Part print with two shaded views. Sizes in mm from the minimum x, y, z corner. Round coordinates to 2 decimals unless told otherwise and drop trailing zeros. Order: outer loops, then holes, each group sorted by start corner. A loop starts at its lowest first (then second) coordinate and runs counter-clockwise, first axis right, second up. Notation, with made-up numbers: (6.5, 40.25) - (45.5, 40.25) arc R16 ccw to (45.5, 51.25) - close; hole circle Ø6 at (65.25, 35). An arc over 180 degrees is marked (long way). Write item = value, one per line.
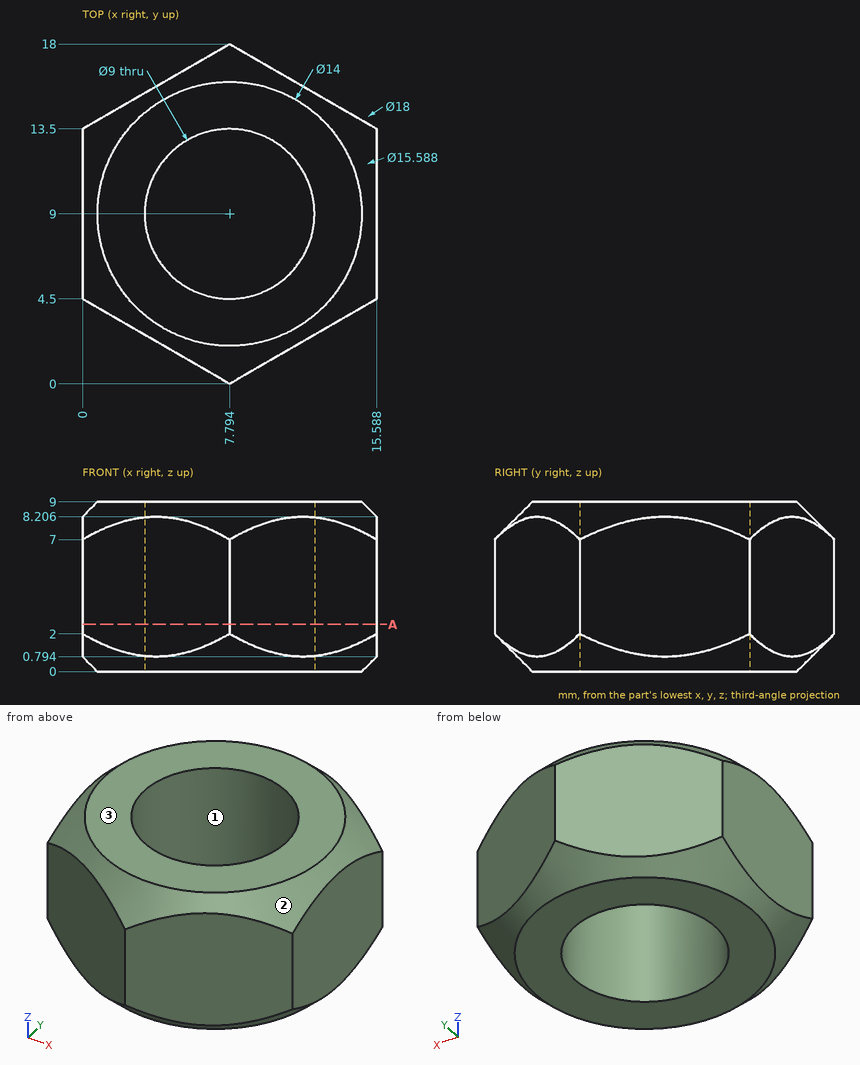
1) Mould opens along Y. For the marked faces 1, 2 and 3 say: +Y half, -Y half, draft (parallel to the pull), parting line (faces both ways), or undercut.
Conclusion:
face_1 = undercut
face_2 = parting line
face_3 = draft
2) Cut at A-A (z = 2.5). Write the cut outline in (x, y) (1 decimal).
Conclusion:
outline = (0, 4.5) - (7.8, 0) - (15.6, 4.5) - (15.6, 13.5) - (7.8, 18) - (0, 13.5) - close; hole circle Ø9 at (7.8, 9)
3) Flat gauge pins, fed straight in: pin 1 Ø1 at (x, z) = (2, 7) entering from -Y; pin 2 Ø2 at (y, z) = (2, 3.5) entering from -X; pin 3 Ø1.5 at (x, z) = (7.5, 1) entering from +Y (1 decimal). Where does each tip first touch, or does it go through?
Conclusion:
pin_1 = 3.06
pin_2 = 2.6
pin_3 = 17.7
4) Wall check: line 1 along X through (y, z) = (9.25, 5.25); line 2 along Y through (x, z) = (5.5, 7.25) (1 decimal); line 3 along Y through (x, z) = (4.75, 3.75) (1 decimal). Give the ranges that are in metal, low to high.
Conclusion:
line_1 = 0 to 3.3, 12.29 to 15.59
line_2 = 1.3 to 5.1, 12.9 to 16.7
line_3 = 1.8 to 5.7, 12.3 to 16.2
